For this review, use the dimensioned drawing (mm, ordinates from the lowest corner) and the shaded views. A direction names the side the tool comes from. Coordinates: 2 decimals unless noted, no trailing zeros. Loops run counter-clockwise (first coordinate to the right, second up) from the corner with the lowest first, then second, coordinate; pieces in that order, holes last. Notation, with made-up numbers: (40, -2) - (92, -2) arc R17 cw to (92, 8) - close; hole circle Ø7 at (45, 49.25). An arc over 180 degrees is marked (long way). Use one line per item in the form item = value. Start each with the question number.
(1) Clearance check with flat-ended pins moving along their axes: pin 1 Ø7 at (x, y) = (24.5, 7.5) entering from +Z; pin 2 Ø4 at (y, z) = (5, 3.5) entering from +X; pin 3 Ø1.5 at (y, z) = (3, 1.5) entering from -X. State where each tip first meets the part, or that it passes through.
(2) Add section D-D (z = 5.25). State the section outline as (x, y) points (1 decimal).
(3) Tool access review of the marked faces 1 and 2: name each direction out of +Z, -Z, +X, -X, +Y, -Y from which nothing blocks a thin tool from reaching the whole face with its end or side.
(4) Add section C-C (y = 8.5). State the section outline as (x, z) points, plus the area to 3 significant figures.
(5) Add section A-A (y = 3). State the section outline as (x, z) points.
(6) The part is to be moulded in two halves that separate along X. For the marked faces 3, 4 and 5, say which applies: pulls with the +X half, pulls with the -X half, needs draft (parallel to the pull), parting line crosses it, or undercut.
(7) For L1, parallel to X at y = 5.25, z = 2.75; L2, parallel to X at y = 5.75, z = 1 (1 decimal); L3, parallel to X at y = 8.25, z = 2.75, list the stretches that pass through material, from the lowest coordinate up.
(8) Add section B-B (z = 3.5). State the section outline as (x, y) points (1 decimal), plus the area to 3 significant figures.
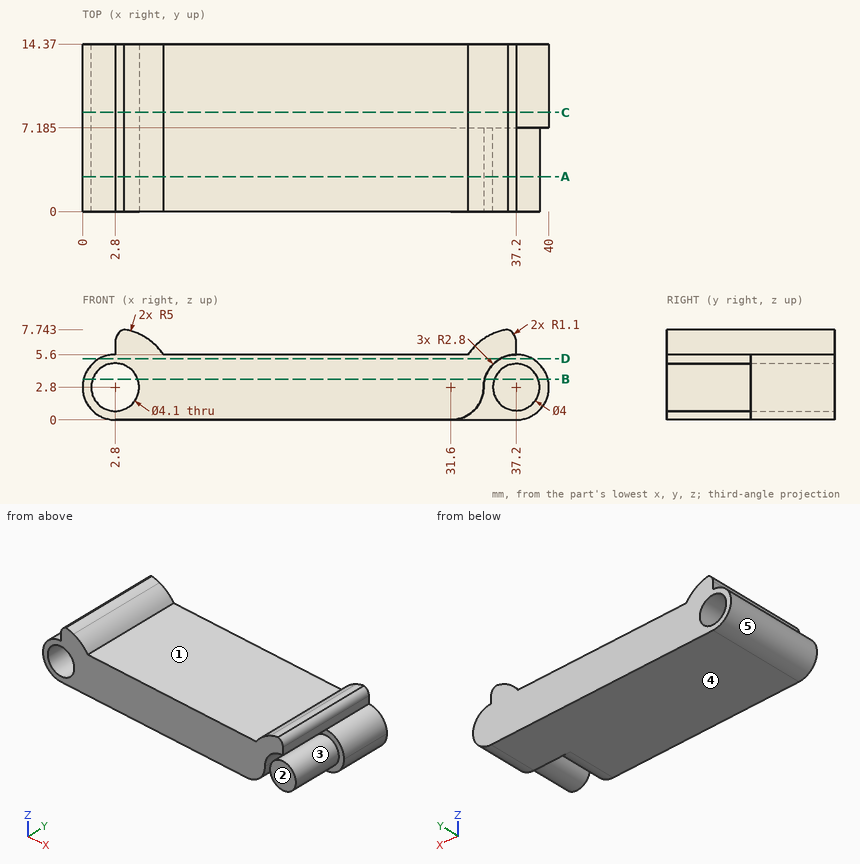
Computed values:
q1.pin_1 = 5.6
q1.pin_2 = 39.2
q1.pin_3 = 0.05
q2.outline = (1.4, 0) - (35.8, 0) - (35.8, 7.2) - (38.6, 7.2) - (38.6, 14.4) - (1.4, 14.4) - close
q3.face_1 = +Z, +Y, -Y
q3.face_2 = +Z, -Z, +X, -X, -Y
q4.outline = (2.8, 0) - (37.2, 0) arc R2.8 ccw to (37.2, 5.6) - (37.2, 6.7) arc R1.1 ccw to (36.45, 7.74) arc R5 ccw to (33.06, 5.6) - (6.94, 5.6) arc R5 ccw to (3.55, 7.74) arc R1.1 ccw to (2.8, 6.7) - (2.8, 5.6) arc R2.8 ccw to start; hole circle Ø4.1 at (2.8, 2.8)
q4.area = 216 mm^2
q5.outline = (2.8, 0) - (31.6, 0) arc R2.8 ccw to (34.4, 2.8) arc R2.8 cw to (37.2, 5.6) - (37.2, 6.7) arc R1.1 ccw to (36.45, 7.74) arc R5 ccw to (33.06, 5.6) - (6.94, 5.6) arc R5 ccw to (3.55, 7.74) arc R1.1 ccw to (2.8, 6.7) - (2.8, 5.6) arc R2.8 ccw to start; circle Ø4 at (37.2, 2.8); hole circle Ø4.1 at (2.8, 2.8)
q6.face_3 = undercut
q6.face_4 = needs draft
q6.face_5 = pulls with the -X half
q7.L1 = 0 to 0.75, 4.85 to 34.4, 35.2 to 39.2
q7.L2 = 0.7 to 1.8, 3.8 to 33.7, 36.3 to 38.1
q7.L3 = 0 to 0.75, 4.85 to 40
q8.outline = (0.1, 0) - (0.9, 0) - (0.9, 14.4) - (0.1, 14.4) - close; (4.7, 0) - (34.5, 0) - (34.5, 7.2) - (35.3, 7.2) - (35.3, 0) - (39.1, 0) - (39.1, 7.2) - (39.9, 7.2) - (39.9, 14.4) - (4.7, 14.4) - close
q8.area = 505 mm^2
